Work out the finished part from the listing and answer in its coordinate system (mm). A direction names the side the tool comes from. Round coordinates to 2 decimals unless told otherwise and drop trailing zeros. Write each loop counter-clockwise with the first axis right and the second up, starting at its lowest first coordinate (ties: lowest second). Pieces come first, ordered by that corner, then holes. Notation, with made-up numbers: (-14.5, 35.5) - (0.5, 35.5) arc R19 ccw to (0.5, 44.5) - close; hole circle Ø11 at (-30, 41.5). An arc over 180 degrees is marked (long way). Answer as a JSON object with one key per item and string values.
```python
from build123d import *

# Parameters (mm, degrees)
SKETCH1_W           = 16
SKETCH1_H           = 12
BOSS_EXTRUDE1_DEPTH = 6.5
CUT_EXTRUDE1_DEPTH  = 12.926860442
SKETCH3_W           = 14
SKETCH3_H           = 7.5
CUT_EXTRUDE2_DEPTH  = 11
SKETCH4_R           = 1.6
CUT_EXTRUDE3_DEPTH  = 16.81929202
FILLET1_R           = 1


with BuildPart() as part:
    # Sketch1 → Boss-Extrude1 (new body)
    with BuildSketch(Plane(origin=(0, 0, 0), x_dir=(0, 0, -1), z_dir=(1, 0, 0))):
        Rectangle(SKETCH1_W, SKETCH1_H)
    extrude(amount=-BOSS_EXTRUDE1_DEPTH)

    # Sketch2 → Cut-Extrude1 (cut, through all)
    with BuildSketch(Plane(origin=(0, 0, 0), x_dir=(0, 0, -1), z_dir=(1, 0, 0))):
        Polygon((8, 0), (2, 6), (8, 6), align=None)
    extrude(amount=-CUT_EXTRUDE1_DEPTH, mode=Mode.SUBTRACT)

    # Sketch3 → Cut-Extrude2 (cut)
    with BuildSketch(Plane.XY.offset(8)):
        with Locations((-3.25, 0)):
            Rectangle(SKETCH3_W, SKETCH3_H)
    extrude(amount=-CUT_EXTRUDE2_DEPTH, mode=Mode.SUBTRACT)

    # Sketch4 → Cut-Extrude3 (cut, through all)
    with BuildSketch(Plane(origin=(0, 6, 0), x_dir=(1, 0, 0), z_dir=(0, 1, 0))):
        with Locations(Location((-3.25, -4.5, 0), (0, 0, 270))):
            Circle(SKETCH4_R)
    extrude(amount=-CUT_EXTRUDE3_DEPTH, mode=Mode.SUBTRACT)

    # Fillet1
    fillet1_edges = [part.edges().sort_by_distance(p)[0] for p in [
        (-3.25, -3.75, -3),
        (-3.25, 3.75, -3),
    ]]
    fillet(fillet1_edges, radius=FILLET1_R)


solid = part.part
```
Item 1: A cutting plane is placed at A-A (x = -3.25). Write down the section's boundary in (y, z).
Results found:
{"outline": "(-6, -8) - (0, -8) - (6, -2) - (6, 2.9) - (3.75, 2.9) - (3.75, -2) arc R1 cw to (2.75, -3) - (-2.75, -3) arc R1 cw to (-3.75, -2) - (-3.75, 2.9) - (-6, 2.9) - close; (-6, 6.1) - (-3.75, 6.1) - (-3.75, 8) - (-6, 8) - close; (3.75, 6.1) - (6, 6.1) - (6, 8) - (3.75, 8) - close"}
Item 2: A cutting plane is placed at C-C (z = 0.25). Write down the section's boundary in (x, y).
Results found:
{"outline": "(-6.5, -6) - (0, -6) - (0, -3.75) - (-6.5, -3.75) - close; (-6.5, 3.75) - (0, 3.75) - (0, 6) - (-6.5, 6) - close"}
Item 3: Consider line 1 along Y through (x, z) = (-3.75, -1); line 2 along X through (y, z) = (4.55, 4.5); line 3 along Z through (x, y) = (-2.75, -1.25). Determine where each line is inside the solid, lowest interval first.
Results found:
{"line 1": "-6 to -3.75, 3.75 to 6", "line 2": "-6.5 to -4.85, -1.65 to 0", "line 3": "-8 to -3"}
Item 4: Determine the mould class of faces 1 (the flat face through (-3, -6, 0)), 2 (the cylindrical face through (-2.769, -4.859, 6.026)), 3 (the flat face through (-3, 5, 8)) for opening direction Z: pulls with the +Z half, pulls with the -Z half, needs draft (parallel to the pull), parting line crosses it, or undercut.
Results found:
{"face 1": "needs draft", "face 2": "undercut", "face 3": "pulls with the +Z half"}
Item 5: For faces 4 (the flat face through (-3, 3, -5)), 5 (the flat face through (-3, 3.75, 2)), determine the directions among +Z, -Z, +X, -X, +Y, -Y from which every point of the face is accessible in a straight line to the end or side of a thin tool.
Results found:
{"face 4": "-Z, +X, -X, +Y", "face 5": "+Z, +X, -X"}
Item 6: A cutting plane is placed at B-B (z = 4.5). Write down the section's boundary in (x, y), and give its area (4 significant figures).
Results found:
{"outline": "(-6.5, -6) - (-4.85, -6) - (-4.85, -3.75) - (-6.5, -3.75) - close; (-6.5, 3.75) - (-4.85, 3.75) - (-4.85, 6) - (-6.5, 6) - close; (-1.65, -6) - (0, -6) - (0, -3.75) - (-1.65, -3.75) - close; (-1.65, 3.75) - (0, 3.75) - (0, 6) - (-1.65, 6) - close", "area": "14.85 mm²"}
Item 7: Each of these flat-tipped pins is pushed along its axis until it touches: P1, Ø2.5, axis at x = -3.25, z = 4.5, coming from the +Y side; P2, Ø1, axis at x = -2.5, z = -3.5, coming from the +Y side. Where does it stop, or does it pass through?
Results found:
{"P1": "through", "P2": "y = 5"}
Item 8: A cutting plane is placed at D-D (y = 5.25). Write down the section's boundary in (x, z), and give its area (3 significant figures).
Results found:
{"outline": "(-6.5, -2.75) - (0, -2.75) - (0, 8) - (-6.5, 8) - close; hole circle Ø3.2 at (-3.25, 4.5)", "area": "61.8 mm²"}
